Source: three-view drawing plus pictorial views. Frame: mm from the lowest corner of the part. A direction names the side the tool comes from. Give positions to 0.01 mm unless a question says otherwise; leave off trailing zeros. Order: outer loops, then holes, each group sorted by start corner. A loop starts at its lowest first (then second) coordinate and runs counter-clockwise, first axis right, second up. Notation, with made-up numbers: M -1,-29.5 L 35,-29.5 A4 cw 35,-24.5 Z; hole C 59,-31.5 d1. An arc over 180 degrees is marked long. One line per question, with ' | ' between items. Start each with the question number.
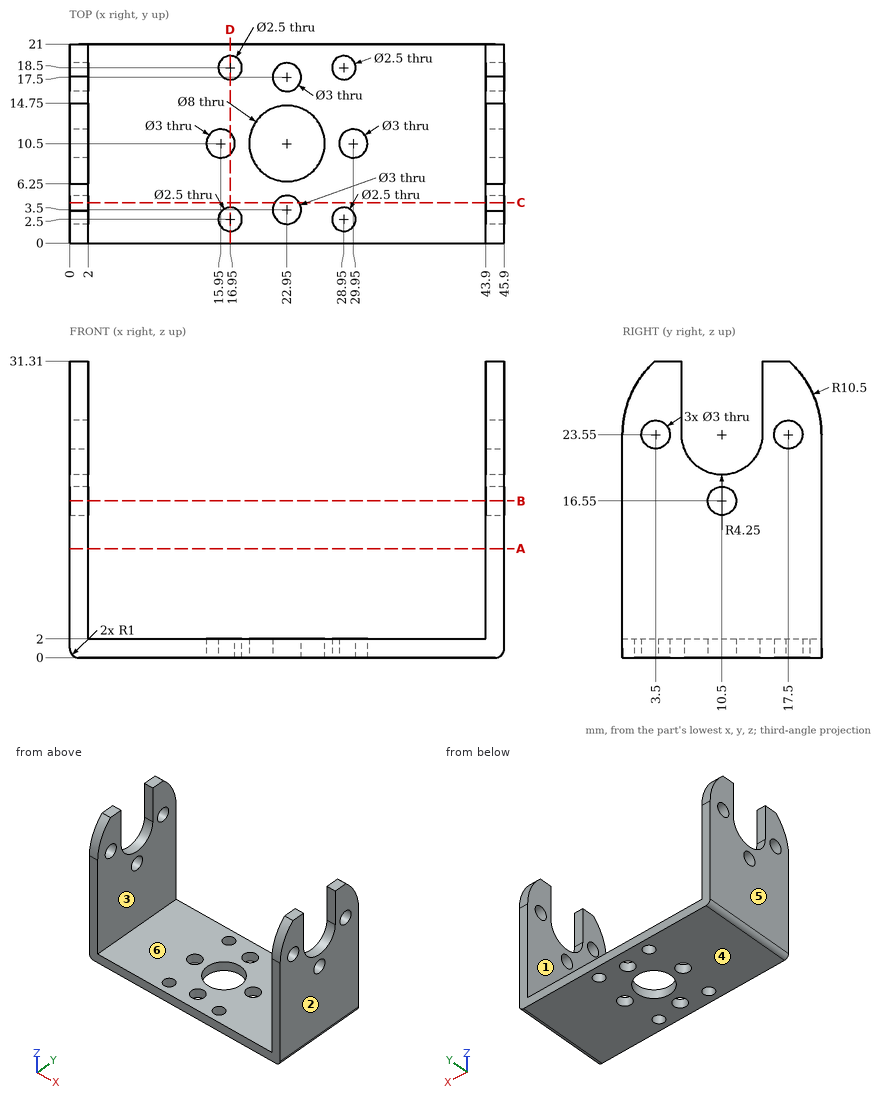
Item 1: Cut plane A-A on z = 11.5. Return the cut outline in (x, y).
Item 2: Line query: line 1 (X direction, y = 3.75, z = 15); line 2 (Y direction, x = 1.65, z = 23.55); line 3 (Y direction, x = 28, z = 1). Output: solid intervals per line, ascending.
Item 3: Mould query, pull axis X, two halves, no side actions, for the marked faces 3, 4, 5 and 6. Classes: pulls with the +X half, pulls with the -X half, needs draft (parallel to the pull), parting line crosses it, or undercut.
Item 4: Cut plane B-B on z = 16.55. Return the cut outline in (x, y).
Item 5: Cut plane D-D on x = 16.95. Return the cut outline in (y, z).
Item 6: Pin query (flat end, axial travel): pin 1 Ø2 at (x, z) = (1, 25.5) entering from -Y; pin 2 Ø1.8 at (y, z) = (10.5, 16.55) entering from +X; pin 3 Ø0.6 at (x, z) = (1, 29) entering from +Y; pin 4 Ø6.5 at (x, y) = (21, 12) entering from +Z. Return the tip coordinate at first contact, or that it passes through.
Item 7: Cut plane C-C on y = 4.25. Return the cut outline in (x, z).
Item 8: Reachability of the marked faces 1 and 2 from +Z, -Z, +X, -X, +Y, -Y: full face, straight path, thin tool, end or side. Return the list, or none.
Results are:
1) outline: M 0,0 L 2,0 L 2,21 L 0,21 Z; M 43.9,0 L 45.9,0 L 45.9,21 L 43.9,21 Z
2) line 1: x = 0 to 2, 43.9 to 45.9 | line 2: y = 0 to 2, 5 to 6.25, 14.75 to 16, 19 to 21 | line 3: y = 0 to 1.69, 3.31 to 17.69, 19.31 to 21
3) face 3: undercut | face 4: needs draft | face 5: pulls with the -X half | face 6: undercut
4) outline: M 0,0 L 2,0 L 2,9 L 0,9 Z; M 0,12 L 2,12 L 2,21 L 0,21 Z; M 43.9,0 L 45.9,0 L 45.9,9 L 43.9,9 Z; M 43.9,12 L 45.9,12 L 45.9,21 L 43.9,21 Z
5) outline: M 0,0 L 1.25,0 L 1.25,2 L 0,2 Z; M 3.75,0 L 9.38,0 L 9.38,2 L 3.75,2 Z; M 11.62,0 L 17.25,0 L 17.25,2 L 11.62,2 Z; M 19.75,0 L 21,0 L 21,2 L 19.75,2 Z
6) pin 1: stops at y = 0.04 | pin 2: passes through | pin 3: stops at y = 19.65 | pin 4: stops at z = 2
7) outline: M 0,1 A1 ccw 1,0 L 21.65,0 L 21.65,2 L 2,2 L 2,22.25 L 0,22.25 Z; M 0,24.85 L 2,24.85 L 2,31.31 L 0,31.31 Z; M 24.25,0 L 44.9,0 A1 ccw 45.9,1 L 45.9,22.25 L 43.9,22.25 L 43.9,2 L 24.25,2 Z; M 43.9,24.85 L 45.9,24.85 L 45.9,31.31 L 43.9,31.31 Z
8) face 1: +Z, +Y, -Y | face 2: +Z, -Z, +X, +Y, -Y
